Geometry check sheet. Reference: the model listing, model coordinates, mm. A direction names the side the tool comes from. Give positions to 0.01 mm unless a question says otherwise; leave off trailing zeros. Write each loop counter-clockwise with the first axis right and the second up, starting at its lowest first coordinate (ties: lowest second). Pieces come first, ordered by that corner, then holes. Notation, with made-up numbers: M 8,44 L 54,44 A13 cw 54,64 Z; hole C 5,17.25 d3. An arc over 180 degrees is marked long. One line per item, written item: value. Start each with the question number.
1. Tool access check on faces 4 (the face through (-0.867, -3.905, 7.395)), 5 (the face through (1, -1, 15)). Record the directions out of +Z, -Z, +X, -X, +Y, -Y that give a thin tool (end or side, any length) a straight path to the whole face; none if there is none.
2. Cross-section at D-D on x = -3.5. Record the cut outline in (y, z).
3. Release check for a two-part mould opening along X. For faces 1 (the face through (0.235, 5.206, -1.972)), 2 (the face through (0, -1, 6)), 3 (the face through (-4.626, -2.399, -1.972)) record: pulls with the +X half, pulls with the -X half, needs draft (parallel to the pull), parting line crosses it, or undercut.
4. Scan lines: line 1 (Y direction, x = 0, z = 7.5); line 2 (Z direction, x = -3, y = -4); line 3 (X direction, y = 1.75, z = 12). Record each from-to range of solid material in increasing order.
5. Gauge pin test, flat ends, axial feed: pin 1 (2 mm diameter, centred on y = -2.5, z = 10.5, fed in from -X); pin 2 (3 mm diameter, centred on x = -2, z = 12, fed in from +Y); pin 3 (1.5 mm diameter, centred on y = -4, z = 5.5, fed in from -X); pin 4 (6 mm diameter, centred on y = 0.5, z = -1, fed in from +X). Record the tip position at first contact, or that the pin passes through.
6. Cross-section at B-B on z = 8.5. Record the cut outline in (x, y), then the cut area to 3 significant figures.
7. Cross-section at C-C on y = -1.75. Record the cut outline in (x, z), then the cut area to 3 significant figures.
8. Cross-section at A-A on x = 0.25. Record the cut outline in (y, z), then the cut area to 3 significant figures.
from build123d import *

# Parameters (mm, degrees)
F0_R      = 4
F1_DEPTH  = 15
F1_FACE_R = 4
F2_DEPTH  = 4
F3_R      = 1
F4_DEPTH  = 19.001


with BuildPart() as f1:
    # F0 (on Top) → F1 (new body)
    with BuildSketch(Plane.XY):
        Circle(F0_R)
    extrude(amount=F1_DEPTH)

    # F1_face (on face) + F0 (on Top) → F2 (join)
    with BuildSketch(Plane(origin=(0, 0, 0), x_dir=(1, 0, 0), z_dir=(0, 0, -1))):
        Circle(F1_FACE_R)
    with BuildSketch(Plane.XY):
        Polygon((6.0127749436, -0.2231464057), (3.1996379279, 5.0956426455), (-2.8131370157, 5.3187890512), (-6.0127749436, 0.2231464057), (-3.1996379279, -5.0956426455), (2.8131370157, -5.3187890512), align=None)
        Circle(F0_R, mode=Mode.SUBTRACT)
    extrude(amount=F2_DEPTH, dir=(0, 0, -1))

    # F3 (on face) → F4 (cut, through all)
    with BuildSketch(Plane.XY.offset(15)):
        Circle(F3_R)
    extrude(amount=-F4_DEPTH, mode=Mode.SUBTRACT)


solid = f1.part
Report:
1. face 4: +Z
1. face 5: +Z, +X, -X, +Y, -Y
2. outline: M -4.53,-4 L 4.22,-4 L 4.22,0 L 1.94,0 L 1.94,15 L -1.94,15 L -1.94,0 L -4.53,0 Z
3. face 1: pulls with the +X half
3. face 2: undercut
3. face 3: pulls with the -X half
4. line 1: y = -4 to -1, 1 to 4
4. line 2: z = -4 to 0
4. line 3: x = -3.6 to 3.6
5. pin 1: stops at x = -3.71
5. pin 2: stops at y = 3.97
5. pin 3: stops at x = -2.33
5. pin 4: stops at x = 6.01
6. outline: C 0,0 d8; hole C 0,0 d2
6. area: 47.1 mm^2
7. outline: M -4.97,-4 L 5.05,-4 L 5.05,0 L 3.6,0 L 3.6,15 L -3.6,15 L -3.6,0 L -4.97,0 Z
7. area: 148 mm^2
8. outline: M -5.22,-4 L -0.97,-4 L -0.97,15 L -3.99,15 L -3.99,0 L -5.22,0 Z; M 0.97,-4 L 5.21,-4 L 5.21,0 L 3.99,0 L 3.99,15 L 0.97,15 Z
8. area: 125 mm^2
